Part model, mm, in its own coordinate system. Face numbers are marked on the shaded views. A direction names the side the tool comes from. Round coordinates to 2 decimals unless told otherwise and drop trailing zeros. Loops run counter-clockwise (first coordinate to the right, second up) from the corner with the lowest first, then second, coordinate; pieces in that order, holes last. Notation, with made-up numbers: (58.25, 28.25) - (109.25, 28.25) arc R19 cw to (109.25, 62.25) - close; hole circle Ø5 at (26, 34). An arc over 180 degrees is marked (long way). Write each question's results on one line, items separated by ' | '. Start each with the question number.
(1) Drill centre lines: L1, parallel to X at y = 15, z = 0; L2, parallel to X at y = 4, z = 20.5. Where is each one in solid material? Low to high.
(2) Flat gauge pins, fed straight in: P1, Ø5, axis at x = 7, z = 12, coming from the +Y side; P2, Ø4, axis at y = 8.5, z = 9.5, coming from the +X side; P3, Ø3.5, axis at x = 15, y = 15, coming from the +Z side; P4, Ø1.9, axis at x = -15, y = -15, coming from the -Z side. Where does each tip first touch, or does it go through?
(3) Mould opens along Y. For the marked faces 1, 2 and 3 say: released by +Y, released by -Y, zero draft, split by the parting line, or undercut.
(4) Tool access for the marked faces 4, 5, 6 and 7: list every direction of +Z, -Z, +X, -X, +Y, -Y with a clear straight run to the whole face (end or side of a thin tool).
(5) Cut at D-D, the plane z = 12.5. List the corners of the cut face in (x, y), then the cut area to 3 significant figures.
(6) Cut at A-A, the plane x = 9.5. List the corners of the cut face in (y, z).
(7) Cut at C-C, the plane x = -15. List the corners of the cut face in (y, z).
Autodesk Inventor part; units mm, degrees
ref_plane "YZ Plane" through (0, 0, 0) normal (1, 0, 0) x (0, 1, 0)
ref_plane "XZ Plane" through (0, 0, 0) normal (0, 1, 0) x (-1, 0, 0)
ref_plane "XY Plane" through (0, 0, 0) normal (0, 0, 1) x (1, 0, 0)
sketch "Sketch1" plane through (0, 0, 0) normal (0, 0, 1) x (1, 0, 0)
  line L0 (-19, 19) -> (19, 19)
  line L1 (19, 19) -> (19, -19)
  line L2 (19, -19) -> (-19, -19)
  line L3 (-19, -19) -> (-19, 19)
  line L4 (-19, 19) -> (19, -19) construction
  line L5 (19, 19) -> (-19, -19) construction
  line L6 (-11, 11) -> (11, 11)
  line L7 (11, 11) -> (11, -11)
  line L8 (11, -11) -> (-11, -11)
  line L9 (-11, -11) -> (-11, 11)
  line L10 (-11, 11) -> (11, -11) construction
  line L11 (11, 11) -> (-11, -11) construction
  point P0 (0, 0)
  dimension "d0" = 38
  dimension "d1" = 38
  dimension "d2" = 22
  dimension "d3" = 22
extrude "Extrusion1" add sketch "Sketch1" along normal mid plane 2
sketch "Sketch2" plane through (0, 0, 1) normal (0, 0, 1) x (1, 0, 0)
  line L0 (-13, 13) -> (13, 13)
  line L1 (13, 13) -> (13, -13)
  line L2 (13, -13) -> (-13, -13)
  line L3 (-13, -13) -> (-13, 13)
  line L4 (-13, 13) -> (13, -13) construction
  line L5 (13, 13) -> (-13, -13) construction
  line L6 (-11, -11) -> (11, -11)
  line L7 (11, -11) -> (11, 11)
  line L8 (11, 11) -> (-11, 11)
  line L9 (-11, 11) -> (-11, -11)
  line L10 (-11, -11) -> (11, 11) construction
  line L11 (11, -11) -> (-11, 11) construction
  point P0 (0, 0)
  dimension "d6" = 26
  dimension "d7" = 26
  dimension "d8" = 22
extrude "Extrusion2" add sketch "Sketch2" along normal blind 40
sketch "Sketch3" plane through (0, 0, -1) normal (0, 0, -1) x (-1, 0, 0)
  line L0 (11, -11) -> (11, 11)
  line L1 (11, 11) -> (-11, 11)
  line L2 (-11, 11) -> (-11, -11)
  line L3 (-11, -11) -> (11, -11)
  line L4 (19, 19) -> (19, -19)
  line L5 (19, -19) -> (-19, -19)
  line L6 (-19, -19) -> (-19, 19)
  line L7 (-19, 19) -> (19, 19)
  point P0 (0, 0)
  point P1 (15, -15)
  point P2 (-15, -15)
  point P3 (15, 15)
  point P4 (-15, 15)
  dimension "d11" = 15
  dimension "d12" = 15
  dimension "d15" = 30
  dimension "d18" = 30
hole "Hole1" at (-15, -15, -1) at (15, -15, -1) at (-15, 15, -1) at (15, 15, -1) direction (0, 0, 1) diameter 3.242 end through all
equation "\"d1\" = d0"
equation "\"d3\" = d2"
equation "\"d7\" = d6"
properties part number "pmtholder"
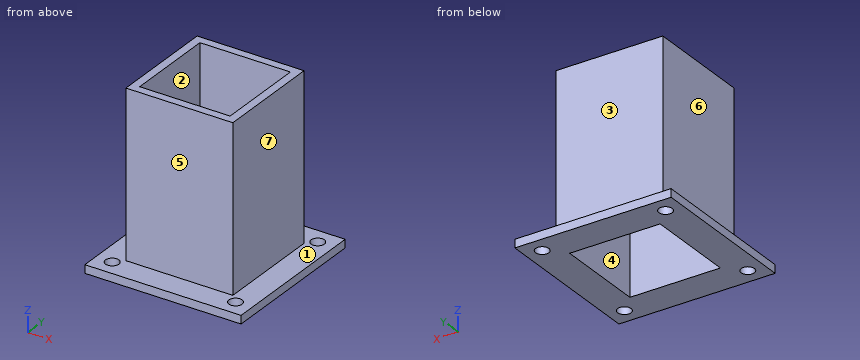
A:
1) L1: -19 to -16.62, -13.38 to 13.38, 16.62 to 19 | L2: -13 to -11, 11 to 13
2) P1: y = 13 | P2: x = 13 | P3: z = 1 | P4: through
3) face 1: zero draft | face 2: undercut | face 3: released by +Y
4) face 4: +Z, -Z | face 5: +Z, +X, -X, -Y | face 6: +Z, -X, +Y, -Y | face 7: +Z, +X, +Y, -Y
5) outline: (-13, -13) - (13, -13) - (13, 13) - (-13, 13) - close; hole (-11, -11) - (11, -11) - (11, 11) - (-11, 11) - close | area: 192 mm2
6) outline: (-19, -1) - (-11, -1) - (-11, 41) - (-13, 41) - (-13, 1) - (-19, 1) - close; (11, -1) - (19, -1) - (19, 1) - (13, 1) - (13, 41) - (11, 41) - close
7) outline: (-19, -1) - (-16.62, -1) - (-16.62, 1) - (-19, 1) - close; (-13.38, -1) - (13.38, -1) - (13.38, 1) - (-13.38, 1) - close; (16.62, -1) - (19, -1) - (19, 1) - (16.62, 1) - close
